For this review, take the finished solid that the model builds, in its own axes (mm). A direction names the side the tool comes from. Coordinates: 2 decimals unless noted, no trailing zeros. Loops run counter-clockwise (first coordinate to the right, second up) from the corner with the lowest first, then second, coordinate; pieces in that order, holes last. Notation, with made-up numbers: (58, 24) - (114, 24) arc R16 cw to (114, 29) - close; hole circle Ø6 at (62.25, 67). An arc over 180 degrees is marked (long way). Answer as a JSON object with one key per item and string values. Group by question number.
Item 1: Tool access review of faces 1 (the flat face through (0, -4, 0.8)), 2 (the flat face through (-1.75, -4.3, 0.5)), 3 (the flat face through (1.75, -4.3, 0.5)), 4 (the flat face through (1.75, 4.2, 0.5)): name each direction out of +Z, -Z, +X, -X, +Y, -Y from which nothing blocks a thin tool from reaching the whole face with its end or side.
Item 2: We need section A-A (x = 0). Give the boundary of the cut face in (y, z) (3 decimals).
Item 3: Mouldability with a two-part tool opening along Z and no side actions: class faces 5 (the flat face through (0, 4, 0.8)), 6 (the flat face through (-1.75, 4.2, 0.5)), 7 (the flat face through (0, 1.6, 0)) as released by +Z, released by -Z, zero draft, split by the parting line, or undercut.
Item 4: We need section B-B (y = 0). Give the boundary of the cut face in (x, z) (3 decimals), then the cut area to 3 significant figures.
Item 5: We need section C-C (z = 0.6). Give the boundary of the cut face in (x, y) (3 decimals), then the cut area to 3 significant figures.
Item 6: We need section D-D (y = 3.5). Give the boundary of the cut face in (x, z).
Item 7: Clearance check with a flat-ended pin moving along its axis: pin 1 (0.5 mm diameter, centred on y = -3.5, z = 0.5, fed in from -X). State where the tip first meets the part, or that it passes through.
Item 8: To check wall thickness, follow line 1 (Y direction, x = 0, z = 0.75) (3 decimals); line 2 (X direction, y = -5, z = 0.45); line 3 (Y direction, x = 0, z = 0.85) (3 decimals). State the ranges of each line that lie inside material, in increasing order.
from build123d import *

# Parameters (mm, degrees)
SKETCH_W        = 3.5
SKETCH_H        = 13.5
PAD_DEPTH       = 0.8
SKETCH003_R     = 2.5
PAD001_DEPTH    = 0.8
SKETCH002_W     = 1
SKETCH002_H     = 3.95
POCKET_DEPTH    = 1.2
SKETCH001_R     = 1.125
POCKET001_DEPTH = 5
SKETCH004_W     = 3.5
SKETCH004_H     = 13.5
PAD002_DEPTH    = 0.2
SKETCH005_R     = 2.5
PAD003_DEPTH    = 0.2
SKETCH006_R     = 1.125
POCKET002_DEPTH = 5


with BuildPart() as part:
    # Sketch → Pad (new body)
    with BuildSketch(Plane.XY):
        Rectangle(SKETCH_W, SKETCH_H)
    extrude(amount=PAD_DEPTH)

    # Sketch003 (on Face6 of Pad) → Pad001 (join)
    with BuildSketch(Plane.XY.offset(0.8)):
        Circle(SKETCH003_R)
    extrude(amount=-PAD001_DEPTH)

    # Sketch002 → Pocket (cut)
    with BuildSketch(Plane.XY.offset(1.3)):
        with Locations((0, 3.975)):
            Rectangle(SKETCH002_W, SKETCH002_H)
        with Locations((0, -3.975)):
            Rectangle(SKETCH002_W, SKETCH002_H)
    extrude(amount=-POCKET_DEPTH, mode=Mode.SUBTRACT)

    # Sketch001 (on Face6 of Pad) → Pocket001 (cut)
    with BuildSketch(Plane.XY.offset(0.8)):
        Circle(SKETCH001_R)
    extrude(amount=-POCKET001_DEPTH, mode=Mode.SUBTRACT)

    # Sketch004 (on Face5 of Pocket001) → Pad002 (join)
    with BuildSketch(Plane.XY.offset(0.8)):
        Rectangle(SKETCH004_W, SKETCH004_H)
    extrude(amount=PAD002_DEPTH)

    # Sketch005 (on Face16 of Pad002) → Pad003 (join)
    with BuildSketch(Plane.XY.offset(0.8)):
        Circle(SKETCH005_R)
    extrude(amount=PAD003_DEPTH)

    # Sketch006 (on Face28 of Pad003) → Pocket002 (cut)
    with BuildSketch(Plane.XY.offset(1)):
        Circle(SKETCH006_R)
    extrude(amount=-POCKET002_DEPTH, mode=Mode.SUBTRACT)


solid = part.part
Check sheet entries:
{
 "1": {"face 1": "none", "face 2": "+Z, -Z, -X, -Y", "face 3": "+Z, -Z, +X, -Y", "face 4": "+Z, -Z, +X, +Y"},
 "2": {"outline": "(-6.75, 0) - (-1.125, 0) - (-1.125, 1) - (-6.75, 1) - close; (1.125, 0) - (6.75, 0) - (6.75, 1) - (1.125, 1) - close; hole (-5.95, 0.1) - (-2, 0.1) - (-2, 0.8) - (-5.95, 0.8) - close; hole (2, 0.1) - (5.95, 0.1) - (5.95, 0.8) - (2, 0.8) - close"},
 "3": {"face 5": "undercut", "face 6": "zero draft", "face 7": "released by -Z"},
 "4": {"outline": "(-2.5, 0) - (-1.125, 0) - (-1.125, 1) - (-2.5, 1) - close; (1.125, 0) - (2.5, 0) - (2.5, 1) - (1.125, 1) - close", "area": "2.75 mm2"},
 "5": {"outline": "(-1.75, -6.75) - (1.75, -6.75) - (1.75, -1.785) arc R2.5 ccw to (1.75, 1.785) - (1.75, 6.75) - (-1.75, 6.75) - (-1.75, 1.785) arc R2.5 ccw to (-1.75, -1.785) - close; hole circle Ø2.25 at (0, 0); hole (-0.5, -5.95) - (0.5, -5.95) - (0.5, -2) - (-0.5, -2) - close; hole (-0.5, 2) - (0.5, 2) - (0.5, 5.95) - (-0.5, 5.95) - close", "area": "39.1 mm2"},
 "6": {"outline": "(-1.75, 0) - (1.75, 0) - (1.75, 1) - (-1.75, 1) - close; hole (-0.5, 0.1) - (0.5, 0.1) - (0.5, 0.8) - (-0.5, 0.8) - close"},
 "7": {"pin 1": "stops at x = -1.75"},
 "8": {"line 1": "y = -6.75 to -5.95, -2 to -1.125, 1.125 to 2, 5.95 to 6.75", "line 2": "x = -1.75 to -0.5, 0.5 to 1.75", "line 3": "y = -6.75 to -1.125, 1.125 to 6.75"}
}
